from build123d import *

# Parameters (mm, degrees)
SKETCH1_R      = 7.7
EXTRUDE1_DEPTH = 2
FILLET1_R      = 0.3
EXTRUDE2_DEPTH = 1.5
FILLET2_R      = 0.3
SKETCH3_R      = 2
EXTRUDE4_DEPTH = 4


with BuildPart() as part:
    # Sketch1 → Extrude1 (new body)
    with BuildSketch(Plane.XY):
        Circle(SKETCH1_R)
    extrude(amount=EXTRUDE1_DEPTH)

    # Fillet1
    fillet1_edges = [part.edges().sort_by_distance(p)[0] for p in [
        (-7.7, 0, 0),
        (-7.7, 0, 2),
    ]]
    fillet(fillet1_edges, radius=FILLET1_R)

    # Sketch2 → Extrude2 (cut)
    with BuildSketch(Plane(origin=(0, 0, 0), x_dir=(-1, 0, 0), z_dir=(0, 0, -1))):
        Polygon((3.049554036, 0), (1.524777018, 2.640991265), (-1.524777018, 2.640991265), (-3.049554036, 0), (-1.524777018, -2.640991265), (1.524777018, -2.640991265), align=None)
    extrude(amount=-EXTRUDE2_DEPTH, mode=Mode.SUBTRACT)

    # Fillet2
    fillet2_edges = [part.edges().sort_by_distance(p)[0] for p in [
        (-2.287165527, -1.320495633, 1.5),
        (-3.049554036, 0, 0.75),
        (0, -2.640991265, 1.5),
        (-1.524777018, -2.640991265, 0.75),
        (2.287165527, -1.320495633, 1.5),
        (1.524777018, -2.640991265, 0.75),
        (2.287165527, 1.320495633, 1.5),
        (3.049554036, 0, 0.75),
        (0, 2.640991265, 1.5),
        (1.524777018, 2.640991265, 0.75),
        (-2.287165527, 1.320495633, 1.5),
        (-1.524777018, 2.640991265, 0.75),
        (-2.287165527, -1.320495633, 0),
        (-2.287165527, 1.320495633, 0),
        (0, 2.640991265, 0),
        (2.287165527, 1.320495633, 0),
        (2.287165527, -1.320495633, 0),
        (0, -2.640991265, 0),
    ]]
    fillet(fillet2_edges, radius=FILLET2_R)

    # Sketch3 → Extrude4 (add)
    with BuildSketch(Plane.XY.offset(2)):
        Circle(SKETCH3_R)
    extrude(amount=EXTRUDE4_DEPTH)


solid = part.part
Could you check a few things on this model? Use its own coordinates, in mm. A direction names the side the tool comes from. Give positions to 0.01 mm unless a question says otherwise; leave off trailing zeros. Write each loop counter-clockwise with the first axis right and the second up, starting at its lowest first coordinate (ties: lowest second). Pieces come first, ordered by that corner, then holes. Notation, with made-up numbers: (61, 80.5) - (88, 80.5) arc R19 ccw to (88, 91.5) - close; hole circle Ø8 at (51.25, 41.5). An arc over 180 degrees is marked (long way). Use CSV: the item, a comma, the result in double quotes. Start each with the question number.
Item 1: If we mould it in two halves opening along Y, with no side actions, what happens to faces 1 (the face through (-1.669, -7.517, 0.99)), 2 (the face through (-0.1, -3.2, 0)), 3 (the face through (2.204, -1.294, 1.41))? For each: pulls with the +Y half, pulls with the -Y half, needs draft (parallel to the pull), parting line crosses it, or undercut.
Item 2: I want a section at B-B, the plane z = 2.9. Please give me the cut outline in (x, y), then the cut area to 3 significant figures.
Item 3: If I drill on line 1 along Z through (x, y) = (-1.75, -4.75); line 2 along Z through (x, y) = (0.5, 0.25); line 3 along X through (y, z) = (2.5, 0.45), over which ranges is the centre line in solid material (lowest first)?
Item 4: For faces 4 (the face through (0, 0, 6)), 5 (the face through (-2.37, -1.35, 0.09)), 6 (the face through (2, -2, 2)), which set-ups out of +Z, -Z, +X, -X, +Y, -Y let a thin tool reach every point of the face, with its end or its side?
Item 5: I'm going to push a flat-ended pin straight in: pin 1 (3 mm diameter, centred on y = 4.5, z = 1.5, fed in from -X). Where does the tip first touch, or does it pass through?
Item 6: I want a section at A-A, the plane x = 0. Please give me the cut outline in (y, z).
Findings:
1,face 1,"parting line crosses it"
1,face 2,"needs draft"
1,face 3,"undercut"
2,outline,"circle Ø4 at (0, 0)"
2,area,"12.6 mm2"
3,line 1,"z = 0 to 2"
3,line 2,"z = 1.5 to 6"
3,line 3,"x = -7.28 to -1.61, 1.61 to 7.28"
4,face 4,"+Z, +X, -X, +Y, -Y"
4,face 5,"-Z"
4,face 6,"+Z"
5,pin 1,"stops at x = -7.09"
6,outline,"(-7.7, 0.3) arc R0.3 ccw to (-7.4, 0) - (-2.94, 0) arc R0.3 ccw to (-2.64, 0.3) - (-2.64, 1.2) arc R0.3 cw to (-2.34, 1.5) - (2.34, 1.5) arc R0.3 cw to (2.64, 1.2) - (2.64, 0.3) arc R0.3 ccw to (2.94, 0) - (7.4, 0) arc R0.3 ccw to (7.7, 0.3) - (7.7, 1.7) arc R0.3 ccw to (7.4, 2) - (2, 2) - (2, 6) - (-2, 6) - (-2, 2) - (-7.4, 2) arc R0.3 ccw to (-7.7, 1.7) - close"
